```python
from build123d import *

# Parameters (mm, degrees)
SKETCH1_R           = 20
BOSS_EXTRUDE1_DEPTH = 50
SKETCH2_R           = 5
BOSS_EXTRUDE2_DEPTH = 10
SKETCH3_R           = 1.5
CUT_EXTRUDE1_DEPTH  = 16
SKETCH4_W           = 49.5
SKETCH4_H           = 49.5
BOSS_EXTRUDE3_DEPTH = 34.75


with BuildPart() as part:
    # Sketch1 → Boss-Extrude1 (new body)
    with BuildSketch(Plane(origin=(0, 0, 0), x_dir=(1, 0, 0), z_dir=(0, 1, 0))):
        with Locations(Location((0, 0, 0), (0, 0, 270))):
            Circle(SKETCH1_R)
    extrude(amount=BOSS_EXTRUDE1_DEPTH)

    # Sketch2 → Boss-Extrude2 (add)
    with BuildSketch(Plane(origin=(0, 50, 0), x_dir=(1, 0, 0), z_dir=(0, 1, 0))):
        with Locations(Location((0, 0, 0), (0, 0, 270))):
            Circle(SKETCH2_R)
    extrude(amount=BOSS_EXTRUDE2_DEPTH)

    # Sketch3 → Cut-Extrude1 (cut)
    with BuildSketch(Plane.XY):
        with Locations((0, 55.836490144)):
            Circle(SKETCH3_R)
    extrude(amount=-CUT_EXTRUDE1_DEPTH, mode=Mode.SUBTRACT)

    # Sketch4 → Boss-Extrude3 (add)
    with BuildSketch(Plane(origin=(0, 0, 0), x_dir=(-1, 0, 0), z_dir=(0, -1, 0))):
        Rectangle(SKETCH4_W, SKETCH4_H)
    extrude(amount=BOSS_EXTRUDE3_DEPTH)


solid = part.part
```
The listing builds one solid part. Answer for the finished solid, in the listing's coordinates (mm). A direction names the side the tool comes from. Coordinates: 2 decimals unless noted, no trailing zeros. Loops run counter-clockwise (first coordinate to the right, second up) from the corner with the lowest first, then second, coordinate; pieces in that order, holes last. Notation, with made-up numbers: (24.25, -28.5) -> (62.25, -28.5) arc R17 cw to (62.25, 1.5) -> close; hole circle Ø4 at (1, 65). An arc over 180 degrees is marked (long way). Use one line per item in the form item = value. Start each with the question number.
Item 1: Consider L1, parallel to Y at x = 0, z = -1.15; L2, parallel to Y at x = -2, z = 19; L3, parallel to Y at x = 23.5, z = 20.5. Determine where each line is inside the solid, lowest interval first. Write a range as [from, to].
Item 2: Flat-ended cylindrical pins translate along their axes: pin 1 Ø1.8 at (x, y) = (0, 55.84) entering from +Z; pin 2 Ø1.5 at (y, z) = (35.5, -14) entering from -X; pin 3 Ø3 at (x, z) = (7.5, -7) entering from +Y. Find the tip coordinate at first contact, or state that the pin passes through.
Item 3: The mould has two halves that part along Y. Classify faces 1 (the face through (-0.195, 57.324, -2.465)), 2 (the face through (11, 0, -17)), 3 (the face through (0, -17, -24.75)): released by +Y, released by -Y, zero draft, split by the parting line, or undercut.
Item 4: The part is cut by section A-A on x = 0. Determine the outline of the cut face in (y, z).
Item 5: The part is cut by section C-C on z = -1. Determine the outline of the cut face in (x, y), then the cut area to 3 significant figures.
Item 6: A tool of negligible diameter and unlimited length cuts with its end or side. For faces 4 (the face through (0, 56, 0)), 5 (the face through (0, -34.75, 0)), 6 (the face through (-19.524, 24.65, -4.336)), from which of +Z, -Z, +X, -X, +Y, -Y can it reach the whole face along a straight path? Write none if from no direction.
Item 7: The part is cut by section B-B on z = 16. Determine the outline of the cut face in (x, y).
Item 8: The part is cut by section D-D on y = 49. Determine the outline of the cut face in (x, z).
Answer key:
q1.L1 = [-34.75, 54.34], [57.34, 60]
q1.L2 = [-34.75, 50]
q1.L3 = [-34.75, 0]
q2.pin_1 = 5
q2.pin_2 = -14.98
q2.pin_3 = 50
q3.face_1 = undercut
q3.face_2 = released by +Y
q3.face_3 = zero draft
q4.outline = (-34.75, -24.75) -> (0, -24.75) -> (0, -20) -> (50, -20) -> (50, -5) -> (54.34, -5) -> (54.34, 0) -> (57.34, 0) -> (57.34, -5) -> (60, -5) -> (60, 5) -> (50, 5) -> (50, 20) -> (0, 20) -> (0, 24.75) -> (-34.75, 24.75) -> close
q5.outline = (-24.75, -34.75) -> (24.75, -34.75) -> (24.75, 0) -> (19.97, 0) -> (19.97, 50) -> (4.9, 50) -> (4.9, 60) -> (-4.9, 60) -> (-4.9, 50) -> (-19.97, 50) -> (-19.97, 0) -> (-24.75, 0) -> close; hole circle Ø3 at (0, 55.84)
q5.area = 3,810 mm2
q6.face_4 = -Z
q6.face_5 = +Z, -Z, +X, -X, -Y
q6.face_6 = +Y
q7.outline = (-24.75, -34.75) -> (24.75, -34.75) -> (24.75, 0) -> (12, 0) -> (12, 50) -> (-12, 50) -> (-12, 0) -> (-24.75, 0) -> close
q8.outline = circle Ø40 at (0, 0)
